Part model, mm, in its own coordinate system. A direction names the side the tool comes from. Give positions to 0.01 mm unless a question says otherwise; leave off trailing zeros. Order: outer loops, then holes, each group sorted by start corner. A loop starts at its lowest first (then second) coordinate and runs counter-clockwise, first axis right, second up. Notation, with made-up numbers: (8.25, 65.5) - (39.25, 65.5) arc R21 cw to (39.25, 80.5) - close; hole circle Ø7 at (4, -8). An arc over 180 degrees is marked (long way). One line per item, written item: value.
```python
from build123d import *

# Parameters (mm, degrees)
F3_DEPTH = 15
F4_R     = 5
F5_DEPTH = 25
F6_SIZE  = 2.5


with BuildPart() as f1:
    # F0 (on Front) → F1 (revolve)
    with BuildSketch(Plane.XZ):
        Polygon((-24.945579, 0), (-0.863729, 0), (-0.863729, 33.33446), (-5.200911, 40.288184), (-20.608397, 40.288184), (-24.945579, 33.33446), align=None)
    revolve(axis=Axis((-33.212595, 0, 0), (-1, 0, 0)))

    # F2 (on face) → F3 (join)
    with BuildSketch(Plane.YZ.offset(-0.863729)):
        Polygon((9.813965, -7.74184), (11.611613, 4.628223), (1.797647, 12.370063), (-9.813965, 7.74184), (-11.611613, -4.628223), (-1.797647, -12.370063), align=None)
    extrude(amount=F3_DEPTH)

    # F4 (on face) → F5 (join)
    with BuildSketch(Plane.YZ.offset(14.136271)):
        Circle(F4_R)
    extrude(amount=F5_DEPTH)

    # F6
    f6_edges = [f1.edges().sort_by_distance(p)[0] for p in [
        (14.136271, 4.008159, -10.055952),
        (14.136271, -4.008159, 10.055952),
    ]]
    chamfer(f6_edges, length=F6_SIZE)


solid = f1.part
```
1) Drop flat-ended pins along their axis: P1, Ø8, axis at x = 11.5, z = -0.5, coming from the +Y side; P2, Ø10, axis at x = 0.5, y = 8, coming from the -Z side; P3, Ø4, axis at x = 27, y = 6.5, coming from the +Z side; P4, Ø17, axis at y = -5, z = -0.5, coming from the +X side. Give the stop position or say it passes through.
Answer:
P1: stops at y = 11.45
P2: stops at z = -38.4
P3: stops at z = 2.18
P4: stops at x = 39.14
2) Slice it at B-B on y = 0. Write the cut outline in (x, z).
Answer:
outline: (-24.95, -33.33) - (-20.61, -40.29) - (-5.2, -40.29) - (-0.86, -33.33) - (-0.86, -11.65) - (11.64, -11.65) - (14.14, -8.96) - (14.14, -5) - (39.14, -5) - (39.14, 5) - (14.14, 5) - (14.14, 8.96) - (11.64, 11.65) - (-0.86, 11.65) - (-0.86, 33.33) - (-5.2, 40.29) - (-20.61, 40.29) - (-24.95, 33.33) - close
3) Slice it at A-A on z = 0. Write the cut outline in (x, y).
Answer:
outline: (-24.95, -33.33) - (-20.61, -40.29) - (-5.2, -40.29) - (-0.86, -33.33) - (-0.86, -10.94) - (14.14, -10.94) - (14.14, -5) - (39.14, -5) - (39.14, 5) - (14.14, 5) - (14.14, 10.94) - (-0.86, 10.94) - (-0.86, 33.33) - (-5.2, 40.29) - (-20.61, 40.29) - (-24.95, 33.33) - close
4) Wall check: line 1 along X through (y, z) = (1.5, -6.5); line 2 along X through (y, z) = (21, -13); line 3 along Y through (x, z) = (-11.5, 1.5). Give the ranges that are in metal, low to high. Write a range as [from, to].
Answer:
line 1: x = [-24.95, 14.14]
line 2: x = [-24.95, -0.86]
line 3: y = [-40.26, 40.26]
5) Which spindle directions (+Z, -Z, +X, -X, +Y, -Y) get a long thin tool onto all of the face, cutting with end or side? Do faces 1 (the face through (6.531, -6.773, -8.445)), 2 (the face through (5.3, 3.9, -10.1)), 3 (the face through (-0.864, 8, 8)), 4 (the face through (5.3, -3.9, 10.1)). Say none if no direction does.
Answer:
face 1: -Z, +X, -Y
face 2: -Z, +X, +Y
face 3: +X
face 4: +Z, +X, -Y
